Design review of the part built by this model. Coordinates are the model's own, in mm. Coordinates: 2 decimals unless noted, no trailing zeros. Write each loop counter-clockwise with the first axis right and the second up, starting at its lowest first coordinate (ties: lowest second). Pieces come first, ordered by that corner, then holes. Notation, with made-up numbers: (-39.75, 23.5) -> (-14.75, 23.5) arc R7 ccw to (-14.75, 34.5) -> close; hole circle Ø10 at (-21, 52.5). An arc over 180 degrees is marked (long way). One line per question, with ' | ' between items. Start each with the question number.
Q1. Add section C-C on x = 18.25. State the section outline as (y, z) points, and give its area (3 significant figures).
Q2. Wall thickness on probe 1 along Z at (x, y) = (2.5, 13); probe 2 along Y at (x, z) = (15, 270.5): over which ranges is each line inside the solid? List them lowest first.
Q3. Add section A-A on y = 11.5. State the section outline as (x, z) points.
Q4. Add section B-B on z = 83. State the section outline as (x, y) points, and give its area (3 significant figures).
Q5. For P1, Ø10, axis at x = 16.5, z = 188.5, coming from the +Y side; P2, Ø3, axis at y = 16.5, z = 58, coming from the +X side, all flat-tipped, find the tip position at first contact; note any pin that passes through.
from build123d import *

# Parameters (mm, degrees)
EXTRUDE_1_DEPTH     = 304.8
SKETCH_2_W          = 167.801792078
SKETCH_2_H          = 21.76
CUT_EXTRUDE_1_DEPTH = 304.8
SKETCH_4_R          = 2.54
CUT_EXTRUDE_2_DEPTH = 304.8


with BuildPart() as part:
    # 草图1 → 凸台-拉伸1 (new body)
    with BuildSketch(Plane.XY):
        Polygon((0, 0), (0, 25), (3.24, 25), (3.24, 3.24), (25, 3.24), (25, 0), align=None)
    extrude(amount=EXTRUDE_1_DEPTH)

    # 草图2 → 切除-拉伸1 (cut)
    with BuildSketch(Plane(origin=(3.24, 0, 0), x_dir=(0, 0, -1), z_dir=(1, 0, 0))):
        with Locations((-156.372580305, 14.12)):
            Rectangle(SKETCH_2_W, SKETCH_2_H)
    extrude(amount=-CUT_EXTRUDE_1_DEPTH, mode=Mode.SUBTRACT)

    # 草图4 → 切除-拉伸2 (cut)
    with BuildSketch(Plane(origin=(0, 3.24, 0), x_dir=(1, 0, 0), z_dir=(0, 1, 0))):
        with Locations(Location((12.797495231, -134.915130156, 0), (0, 0, 270))):
            Circle(SKETCH_4_R)
        with Locations(Location((12.803446161, -185.715129807, 0), (0, 0, 270))):
            Circle(SKETCH_4_R)
    extrude(amount=-CUT_EXTRUDE_2_DEPTH, mode=Mode.SUBTRACT)


solid = part.part
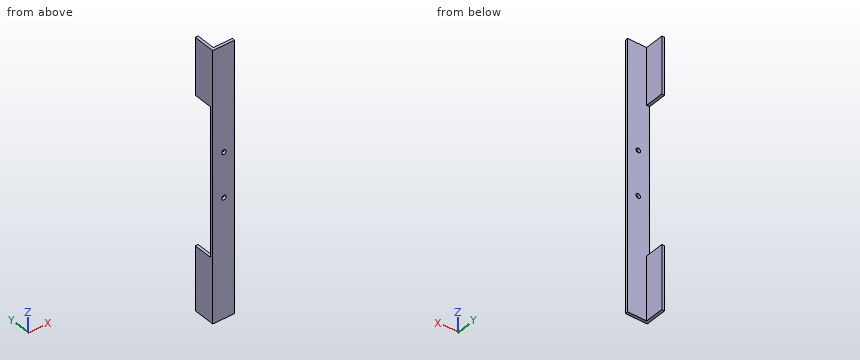
Output values:
1) outline: (0, 0) -> (3.24, 0) -> (3.24, 304.8) -> (0, 304.8) -> close | area: 988 mm2
2) probe 1: z = 0 to 72.47, 240.27 to 304.8 | probe 2: y = 0 to 3.24
3) outline: (0, 0) -> (3.24, 0) -> (3.24, 72.47) -> (0, 72.47) -> close; (0, 240.27) -> (3.24, 240.27) -> (3.24, 304.8) -> (0, 304.8) -> close
4) outline: (0, 0) -> (25, 0) -> (25, 3.24) -> (0, 3.24) -> close | area: 81.0 mm2
5) P1: stops at y = 3.24 | P2: stops at x = 3.24
